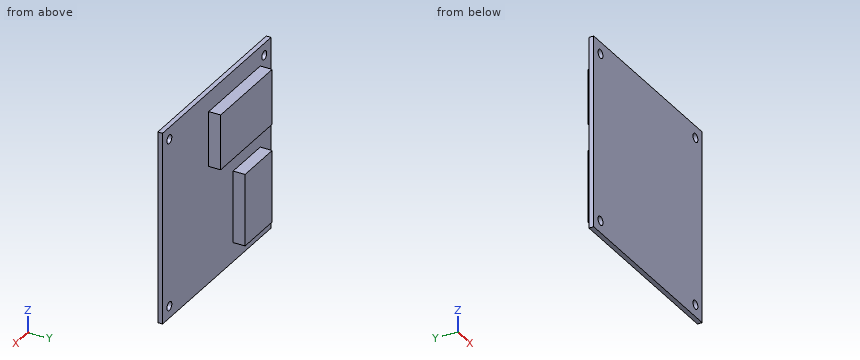
from build123d import *

# Parameters (mm, degrees)
SKETCH1_W              = 80
SKETCH1_H              = 80
PCB_DEPTH              = 2
SKETCH2_R              = 1.8
ATTACHMENT_HOLES_DEPTH = 3
LPATTERN1_COUNT        = 2
LPATTERN1_PITCH        = 70
LPATTERN1_COUNT_DIR2   = 2
LPATTERN1_PITCH_DIR2   = 70
SKETCH3_W              = 20
SKETCH3_H              = 30
GPS_DEPTH              = 5
SKETCH4_W              = 38
SKETCH4_H              = 23
IMU_DEPTH              = 5


with BuildPart() as part:
    # Sketch1 → PCB (new body)
    with BuildSketch(Plane(origin=(0, 0, 0), x_dir=(1, 0, 0), z_dir=(0, 1, 0))):
        with Locations((40, 40)):
            Rectangle(SKETCH1_W, SKETCH1_H)
    extrude(amount=PCB_DEPTH)

    # Sketch2 → Attachment Holes (cut, through all)
    with BuildSketch(Plane(origin=(0, 2, 0), x_dir=(1, 0, 0), z_dir=(0, 1, 0))):
        with Locations((5, 75)):
            Circle(SKETCH2_R)
    attachment_holes = extrude(amount=-ATTACHMENT_HOLES_DEPTH, mode=Mode.SUBTRACT)

    # LPattern1: Attachment Holes 2 × 2
    with Locations(*[(i * LPATTERN1_PITCH, 0, j * LPATTERN1_PITCH_DIR2) for i in range(LPATTERN1_COUNT) for j in range(LPATTERN1_COUNT_DIR2) if (i, j) != (0, 0)]):
        add(attachment_holes, mode=Mode.SUBTRACT)

    # Sketch3 → GPS (add)
    with BuildSketch(Plane(origin=(0, 2, 0), x_dir=(1, 0, 0), z_dir=(0, 1, 0))):
        with Locations((18, 57)):
            Rectangle(SKETCH3_W, SKETCH3_H)
    extrude(amount=GPS_DEPTH)

    # Sketch4 → IMU (add)
    with BuildSketch(Plane(origin=(0, 2, 0), x_dir=(1, 0, 0), z_dir=(0, 1, 0))):
        with Locations((27, 19.5)):
            Rectangle(SKETCH4_W, SKETCH4_H)
    extrude(amount=IMU_DEPTH)


solid = part.part
The listing builds one solid part. Answer for the finished solid, in the listing's coordinates (mm). Round coordinates to 2 decimals unless told otherwise and drop trailing zeros. Order: outer loops, then holes, each group sorted by start corner. A loop starts at its lowest first (then second) coordinate and runs counter-clockwise, first axis right, second up. Notation, with made-up numbers: (-10, 60.25) -> (-6, 60.25) arc R31 cw to (-6, 89.25) -> close; hole circle Ø11 at (-14, -34.75). An arc over 180 degrees is marked (long way). Write each question's results on one line, items separated by ' | '. Start each with the question number.
Q1. Each of these flat-tipped pins is pushed along its axis until it touches: pin 1 (2.5 mm diameter, centred on y = 4, z = -53, fed in from -X); pin 2 (2 mm diameter, centred on x = 34, y = 5, fed in from -Z); pin 3 (2.5 mm diameter, centred on x = 18.5, y = 4, fed in from -Z); pin 4 (3 mm diameter, centred on x = 75, z = -75, fed in from +Y). Where does it stop, or does it pass through?
Q2. Straight lines are drawn through the part: probe 1 along Z at (x, y) = (75, 0.75); probe 2 along X at (y, z) = (0.75, -75); probe 3 along Z at (x, y) = (10.5, 3.5). For each, find the intervals that lie inside material, in ascending order. Write a range as from..to.
Q3. Find section A-A (y = 3.5). Determine the outline of the cut face in (x, z), then the cut area to 3 significant figures.
Q4. Find section B-B (z = -5). Determine the outline of the cut face in (x, y).
Q5. Find section C-C (x = 5). Determine the outline of the cut face in (y, z), then the cut area to 3 significant figures.
Q6. Find section D-D (z = -63.5). Determine the outline of the cut face in (x, y).
Worked answers:
1) pin 1: stops at x = 8 | pin 2: stops at z = -31 | pin 3: stops at z = -72 | pin 4: passes through
2) probe 1: z = -80..-76.8, -73.2..-6.8, -3.2..0 | probe 2: x = 0..3.2, 6.8..73.2, 76.8..80 | probe 3: z = -72..-42, -31..-8
3) outline: (8, -72) -> (28, -72) -> (28, -42) -> (8, -42) -> close; (8, -31) -> (46, -31) -> (46, -8) -> (8, -8) -> close | area: 1,470 mm2
4) outline: (0, 0) -> (3.2, 0) -> (3.2, 2) -> (0, 2) -> close; (6.8, 0) -> (73.2, 0) -> (73.2, 2) -> (6.8, 2) -> close; (76.8, 0) -> (80, 0) -> (80, 2) -> (76.8, 2) -> close
5) outline: (0, -80) -> (2, -80) -> (2, -76.8) -> (0, -76.8) -> close; (0, -73.2) -> (2, -73.2) -> (2, -6.8) -> (0, -6.8) -> close; (0, -3.2) -> (2, -3.2) -> (2, 0) -> (0, 0) -> close | area: 146 mm2
6) outline: (0, 0) -> (80, 0) -> (80, 2) -> (28, 2) -> (28, 7) -> (8, 7) -> (8, 2) -> (0, 2) -> close
